Can you work these out from the drawing? Everything is in mm from the part's minimum corner. A direction names the side the tool comes from. Coordinates: 2 decimals unless noted, no trailing zeros. Write each loop counter-clockwise with the first axis right and the second up, starting at its lowest first coordinate (ties: lowest second). Pieces come first, ordered by that corner, then holes. Notation, with made-up numbers: M 57.25,33.5 L 99.25,33.5 A27 cw 99.25,64.5 Z; hole C -39.75,61.25 d4. An arc over 180 degrees is marked long. Use one line per item in the form item = value. Start each with the question number.
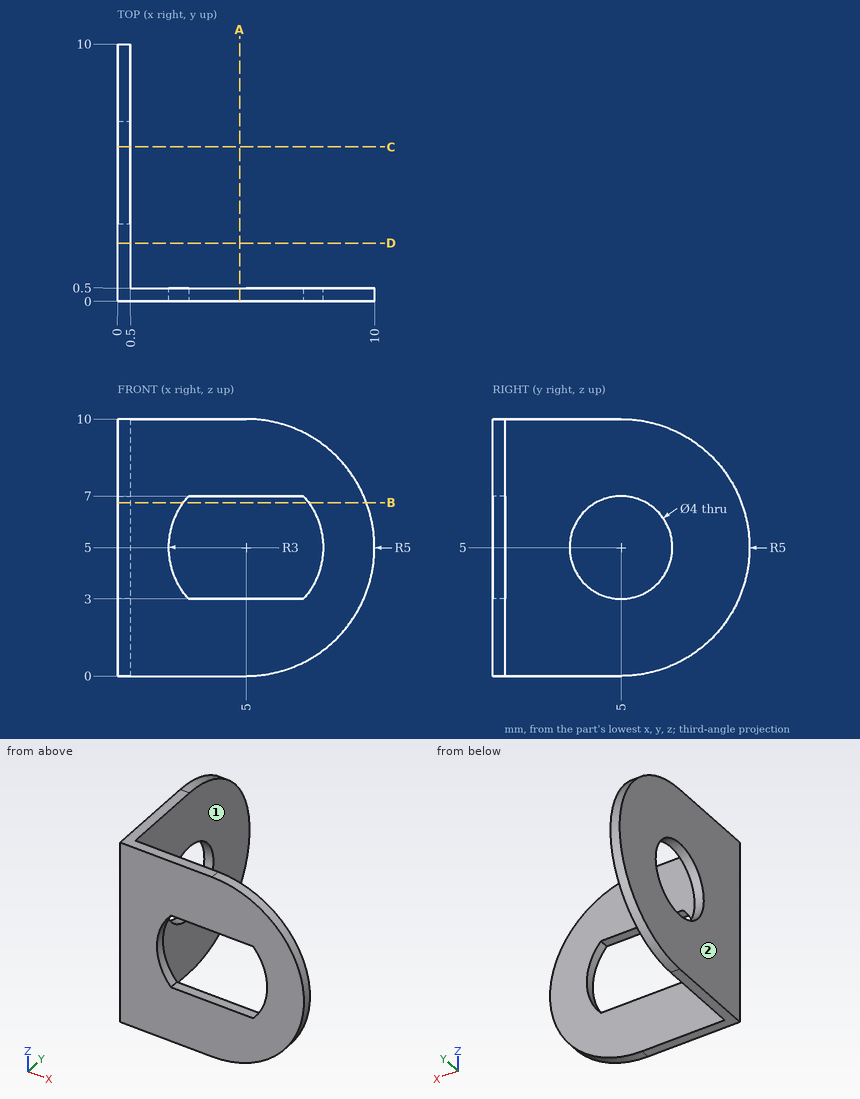
1) Suppose I cut it at A-A on x = 4.75. Please give me the cut outline in (y, z), and give its area (3 significant figures).
2) Suppose I cut it at B-B on z = 6.75. Please give me the cut outline in (x, y), and give its area (3 significant figures).
3) Suppose I cut it at C-C on y = 6. Please give me the cut outline in (x, z), and give its area (3 significant figures).
4) Will these pins go through, and if not, where does the flat tip stop? pin 1 Ø5 at (x, y) = (4.5, 6) entering from +Z; pin 2 Ø5 at (y, z) = (5.5, 3.5) entering from +X.
5) Please list where these lines run through material, in increasing order: line 1 (Y direction, x = 0.4, z = 5); line 2 (X direction, y = 9.25, z = 2.75).
6) Suppose I cut it at D-D on y = 2.25. Please give me the cut outline in (x, z).
7) Which directions (+Z, -Z, +X, -X, +Y, -Y) give clear straight access to the entire face, cutting with the end or side of a thin tool? Please do the marked faces 1 and 2.
Computed values:
q1.outline = M 0,0 L 0.5,0 L 0.5,3 L 0,3 Z; M 0,7 L 0.5,7 L 0.5,10 L 0,10 Z
q1.area = 3.00 mm²
q2.outline = M 0,0 L 2.56,0 L 2.56,0.5 L 0.5,0.5 L 0.5,4.03 L 0,4.03 Z; M 0,5.97 L 0.5,5.97 L 0.5,9.68 L 0,9.68 Z; M 7.44,0 L 9.68,0 L 9.68,0.5 L 7.44,0.5 Z
q2.area = 6.03 mm²
q3.outline = M 0,0.1 L 0.5,0.1 L 0.5,3.27 L 0,3.27 Z; M 0,6.73 L 0.5,6.73 L 0.5,9.9 L 0,9.9 Z
q3.area = 3.17 mm²
q4.pin_1 = through
q4.pin_2 = 0.5
q5.line_1 = 0 to 3, 7 to 10
q5.line_2 = 0 to 0.5
q6.outline = M 0,0 L 0.5,0 L 0.5,10 L 0,10 Z
q7.face_1 = +Z, -Z, +X, +Y
q7.face_2 = +Z, -Z, -X, +Y, -Y
